Autodesk Inventor part; units mm, degrees
ref_plane "YZ Plane" through (0, 0, 0) normal (1, 0, 0) x (0, 1, 0)
ref_plane "XZ Plane" through (0, 0, 0) normal (0, 1, 0) x (-1, 0, 0)
ref_plane "XY Plane" through (0, 0, 0) normal (0, 0, 1) x (1, 0, 0)
sketch "Эскиз1" plane through (0, 0, 0) normal (0, 1, 0) x (-1, 0, 0)
  circle A0 centre (0, 0) radius 4.5
  dimension "d0" = 9
sketch "Эскиз5" plane through (0, 0, 0) normal (0, 1, 0) x (-1, 0, 0)
  point P0 (0, 0)
extrude "Выдавливание4" add sketch "Эскиз1" along normal blind 5
sketch "Эскиз6" plane through (0, 5, 0) normal (0, 1, 0) x (1, 0, 0)
  circle A0 centre (0, 0) radius 4.5
  circle A1 centre (0, 0) radius 1.5
  dimension "d12" = 3
extrude "Выдавливание5" add sketch "Эскиз6" along normal blind 2.5 contours A1
sketch "Эскиз7" plane through (0, 7.5, 0) normal (0, 1, 0) x (1, 0, 0)
  circle A0 centre (0, 0) radius 4.5
  dimension "d15" = 9
extrude "Выдавливание6" add sketch "Эскиз7" along normal blind 55
sketch "Эскиз8" plane through (0, 62.5, 0) normal (0, 1, 0) x (1, 0, 0)
  line L0 (0, 0) -> (0, -2)
  line L1 (0, -2) -> (-5.0098, -2)
  line L2 (0, -2) -> (5.0098, -2)
  line L3 (5.0098, -2) -> (5.0098, -6.5905)
  line L4 (5.0098, -6.5905) -> (-5.0098, -6.5905)
  line L5 (-5.0098, -6.5905) -> (-5.0098, -2)
  dimension "d18" = 2
sketch "Эскиз9" plane through (0, 62.5, 0) normal (0, 1, 0) x (1, 0, 0)
  point P0 (0, 0)
extrude "Выдавливание7" cut sketch "Эскиз8" against normal blind 10
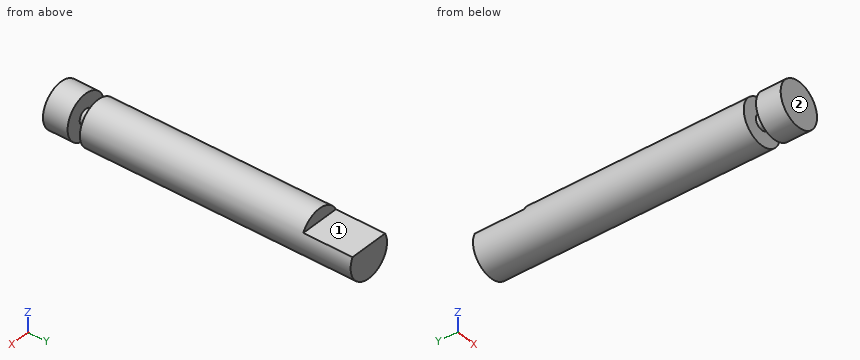
Part model, mm, in its own coordinate system. Face numbers are marked on the shaded views. A direction names the side the tool comes from. Round coordinates to 2 decimals unless told otherwise and drop trailing zeros. Loops run counter-clockwise (first coordinate to the right, second up) from the corner with the lowest first, then second, coordinate; pieces in that order, holes last.
Item 1: Drop flat-ended pins along their axis: P1, Ø3, axis at x = -2.5, y = 43, coming from the -Z side; P2, Ø4, axis at x = 1, y = 59, coming from the +Z side. Give the stop position or say it passes through.
Item 2: 3-axis set-ups, long thin cutter, end or side, ignore diameter. For the marked faces 1 and 2: which of +Z, -Z, +X, -X, +Y, -Y reach the whole face in a straight line?
Item 3: Cut at B-B, the plane x = 0. Give the cut face in (y, z), then the cut area to 4 significant figures.
Item 4: Drill centre lines: line 1 (Y direction, x = -2, z = 3.25); line 2 (Y direction, x = 1.75, z = -3.75); line 3 (Z direction, x = -2, y = 11). Where is each one in solid material? Low to high.
Item 5: Cut at C-C, the plane y = 16.5. Give the cut face in (x, z), then the cut area to 3 significant figures.
Item 6: Cut at A-A, the plane x = -2.25. Give the cut face in (y, z).
A:
1. P1: stops at z = -4.39
1. P2: stops at z = 2
2. face 1: +Z, +X, -X, +Y
2. face 2: +Z, -Z, +X, -X, -Y
3. outline: (0, -4.5) - (5, -4.5) - (5, -1.5) - (7.5, -1.5) - (7.5, -4.5) - (62.5, -4.5) - (62.5, 2) - (52.5, 2) - (52.5, 4.5) - (7.5, 4.5) - (7.5, 1.5) - (5, 1.5) - (5, 4.5) - (0, 4.5) - close
3. area: 522.5 mm2
4. line 1: y = 0 to 5, 7.5 to 52.5
4. line 2: y = 0 to 5, 7.5 to 62.5
4. line 3: z = -4.03 to 4.03
5. outline: circle Ø9 at (0, 0)
5. area: 63.6 mm2
6. outline: (0, -3.9) - (5, -3.9) - (5, 3.9) - (0, 3.9) - close; (7.5, -3.9) - (62.5, -3.9) - (62.5, 2) - (52.5, 2) - (52.5, 3.9) - (7.5, 3.9) - close
